Here's the drawing with two shaded views (mm, measured from the low corner). I have some questions. Round coordinates to 2 decimals unless told otherwise and drop trailing zeros. Order: outer loops, then holes, each group sorted by start corner. A loop starts at its lowest first (then second) coordinate and runs counter-clockwise, first axis right, second up. Notation, with made-up numbers: (89.5, 15.25) - (137.5, 15.25) arc R26 cw to (137.5, 53.25) - close; hole circle Ø10 at (44, 21.25). An arc over 180 degrees is marked (long way). One line per item, written item: value.
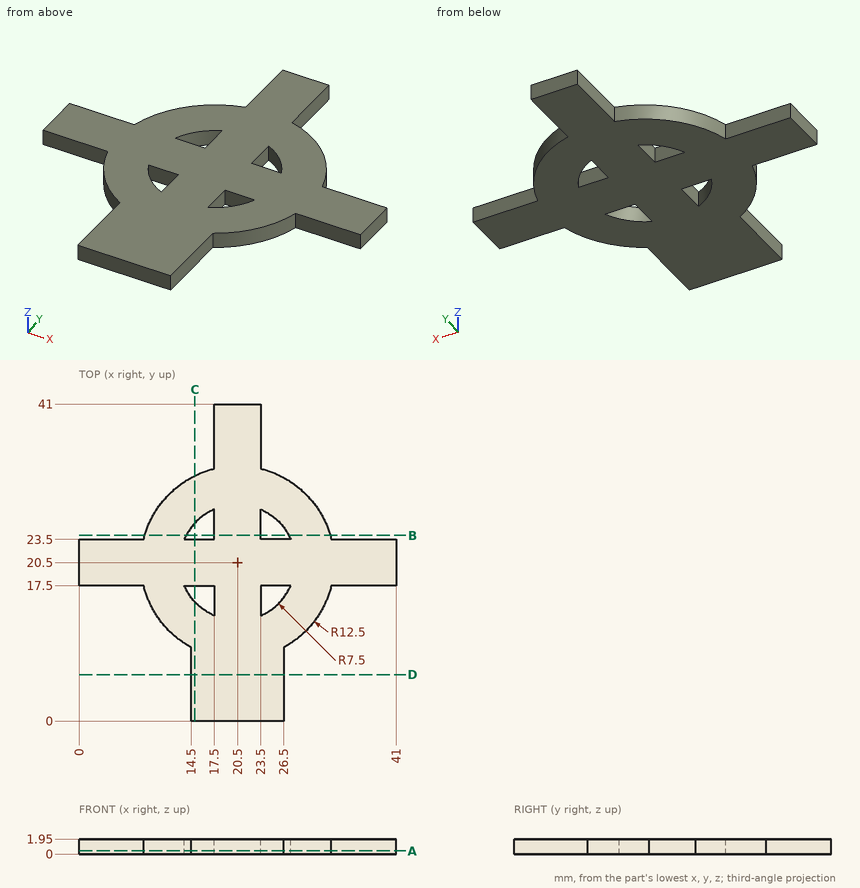
Q1. If we section it at B-B, the plane y = 24: Please give me the cut outline in (x, z).
Results list:
outline: (8.5, 0) - (13.87, 0) - (13.87, 1.95) - (8.5, 1.95) - close; (17.5, 0) - (23.5, 0) - (23.5, 1.95) - (17.5, 1.95) - close; (27.13, 0) - (32.5, 0) - (32.5, 1.95) - (27.13, 1.95) - close
Q2. If we section it at D-D, the plane y = 6: Please give me the cut outline in (x, z), then the cut area to 3 significant figures.
Results list:
outline: (14.5, 0) - (26.5, 0) - (26.5, 1.95) - (14.5, 1.95) - close
area: 23.4 mm²
Q3. If we section it at C-C, the plane x = 15: Please give me the cut outline in (y, z).
Results list:
outline: (0, 0) - (15.4, 0) - (15.4, 1.95) - (0, 1.95) - close; (17.5, 0) - (23.5, 0) - (23.5, 1.95) - (17.5, 1.95) - close; (25.6, 0) - (31.72, 0) - (31.72, 1.95) - (25.6, 1.95) - close
Q4. If we section it at A-A, the plane z = 0.4: Please give me the cut outline in (x, y), then the cut area to 3 significant figures.
Results list:
outline: (0, 17.5) - (8.37, 17.5) arc R12.5 ccw to (14.5, 9.53) - (14.5, 0) - (26.5, 0) - (26.5, 9.53) arc R12.5 ccw to (32.63, 17.5) - (41, 17.5) - (41, 23.5) - (32.63, 23.5) arc R12.5 ccw to (23.5, 32.63) - (23.5, 41) - (17.5, 41) - (17.5, 32.63) arc R12.5 ccw to (8.37, 23.5) - (0, 23.5) - close; hole (13.63, 17.5) arc R7.5 ccw to (17.5, 13.63) - (17.5, 17.5) - close; hole (13.63, 23.5) - (17.5, 23.5) - (17.5, 27.37) arc R7.5 ccw to start; hole (23.5, 13.63) arc R7.5 ccw to (27.37, 17.5) - (23.5, 17.5) - close; hole (23.5, 23.5) - (27.37, 23.5) arc R7.5 ccw to (23.5, 27.37) - close
area: 701 mm²
Q5. If I drill on line 1 along X through (y, z) = (16, 1); line 2 along Y through (x, z) = (27, 0.75); line 3 along Y through (x, z) = (17, 0.65), over which ranges is the centre line in solid material (lowest first)?
Results list:
line 1: 8.84 to 14.5, 17.5 to 23.5, 26.5 to 32.16
line 2: 9.82 to 16.76, 17.5 to 23.5, 24.24 to 31.18
line 3: 0 to 13.87, 17.5 to 23.5, 27.13 to 32.5
Q6. Will these pins go through, and if not, where does the flat tip stop? pin 1 (1 mm diameter, centred on x = 14.5, z = 0.5, fed in from +Y) (3 decimals); pin 2 (1 mm diameter, centred on y = 15, z = 1.5, fed in from -X); pin 3 (1 mm diameter, centred on x = 4.5, z = 1.5, fed in from -Y).
Results list:
pin 1: y = 31.725
pin 2: x = 9.04
pin 3: y = 17.5
